from build123d import *

# Parameters (mm, degrees)
SKETCH8_R           = 1.6
SKETCH8_W           = 27.014473095
SKETCH8_H           = 14.822230288
SKETCH8_R_2         = 2.2
BOSS_EXTRUDE4_DEPTH = 8
SKETCH13_R          = 1.6
BOSS_EXTRUDE5_DEPTH = 3
CHAMFER1_SIZE       = 1
CHAMFER2_SIZE       = 0.5
CHAMFER3_SIZE       = 0.5
SKETCH14_W          = 50
SKETCH14_H          = 36
CUT_EXTRUDE1_DEPTH  = 6
CUT_EXTRUDE2_DEPTH  = 26


with BuildPart() as part:
    # Sketch8 → Boss-Extrude4 (new body)
    with BuildSketch(Plane(origin=(0, 0, 0), x_dir=(1, 0, 0), z_dir=(0, 1, 0))):
        with BuildLine():
            Line((57.021874501, 46.194423092), (3.021874501, 46.194423092))
            ThreePointArc((3.021874501, 46.194423092), (0.900554158, 45.315743435), (0.021874501, 43.194423092))
            Line((0.021874501, 43.194423092), (0.021874501, 3.194423092))
            ThreePointArc((0.021874501, 3.194423092), (0.900554158, 1.073102748), (3.021874501, 0.194423092))
            Line((3.021874501, 0.194423092), (57.021874501, 0.194423092))
            ThreePointArc((57.021874501, 0.194423092), (59.143194845, 1.073102748), (60.021874501, 3.194423092))
            Line((60.021874501, 3.194423092), (60.021874501, 43.194423092))
            ThreePointArc((60.021874501, 43.194423092), (59.143194845, 45.315743435), (57.021874501, 46.194423092))
        make_face()
        with Locations((30.021874501, 2.694423092)):
            Circle(SKETCH8_R, mode=Mode.SUBTRACT)
        with Locations((2.521874501, 23.194423092)):
            Circle(SKETCH8_R, mode=Mode.SUBTRACT)
        with Locations((30.021874501, 43.694423092)):
            Circle(SKETCH8_R, mode=Mode.SUBTRACT)
        Polygon((8.193945871, 28.957965299), (8.193945871, 41.194423092), (51.724223397, 41.194423092), (51.724223397, 37.388033247), (26.110307843, 37.388033247), (26.110307843, 28.957965299), align=None, mode=Mode.SUBTRACT)
        with Locations((41.514637954, 25.761884129)):
            Rectangle(SKETCH8_W, SKETCH8_H, mode=Mode.SUBTRACT)
        with Locations((22.240201254, 24.607965299)):
            Circle(SKETCH8_R_2, mode=Mode.SUBTRACT)
        with Locations((12.021874501, 24.607965299)):
            Circle(SKETCH8_R_2, mode=Mode.SUBTRACT)
    extrude(amount=BOSS_EXTRUDE4_DEPTH)

    # Sketch13 → Boss-Extrude5 (add)
    with BuildSketch(Plane(origin=(0, 8, 0), x_dir=(1, 0, 0), z_dir=(0, 1, 0))):
        with Locations((2.521874501, 23.194423092)):
            Circle(SKETCH13_R)
        with Locations((30.021874501, 2.694423092)):
            Circle(SKETCH13_R)
        with Locations((30.021874501, 43.694423092)):
            Circle(SKETCH13_R)
    extrude(amount=-BOSS_EXTRUDE5_DEPTH)

    # Chamfer1
    chamfer1_edges = [part.edges().sort_by_distance(p)[0] for p in [
        (59.143194845, 8, -1.073102748),
        (60.021874501, 8, -23.194423092),
        (59.143194845, 8, -45.315743435),
        (30.021874501, 8, -46.194423092),
        (0.900554158, 8, -45.315743435),
        (0.021874501, 8, -23.194423092),
        (0.900554158, 8, -1.073102748),
        (30.021874501, 8, -0.194423092),
    ]]
    chamfer(chamfer1_edges, length=CHAMFER1_SIZE)

    # Chamfer2
    chamfer2_edges = [part.edges().sort_by_distance(p)[0] for p in [
        (41.514637954, 8, -33.172999273),
        (55.021874501, 8, -25.761884129),
        (41.514637954, 8, -18.350768985),
        (28.007401406, 8, -25.761884129),
    ]]
    chamfer(chamfer2_edges, length=CHAMFER2_SIZE)

    # Chamfer3
    chamfer3_edges = [part.edges().sort_by_distance(p)[0] for p in [
        (20.040201254, 8, -24.607965299),
        (9.821874501, 8, -24.607965299),
    ]]
    chamfer(chamfer3_edges, length=CHAMFER3_SIZE)

    # Sketch14 → Cut-Extrude1 (cut)
    with BuildSketch(Plane.XZ):
        with Locations((30.021874501, -23.194423092)):
            Rectangle(SKETCH14_W, SKETCH14_H)
    extrude(amount=-CUT_EXTRUDE1_DEPTH, mode=Mode.SUBTRACT)

    # Sketch15 → Cut-Extrude2 (cut)
    with BuildSketch(Plane.ZY.offset(-26.110307843)):
        Polygon((-37.388033247, 7), (-34.086693064, 6), (-37.388033247, 6), align=None)
    extrude(amount=-CUT_EXTRUDE2_DEPTH, mode=Mode.SUBTRACT)


solid = part.part
The model under review builds one solid part; all positions refer to its coordinate system, in mm. A direction names the side the tool comes from. Round coordinates to 2 decimals unless told otherwise and drop trailing zeros. Loops run counter-clockwise (first coordinate to the right, second up) from the corner with the lowest first, then second, coordinate; pieces in that order, holes last. Notation, with made-up numbers: M 40.5,17 L 86.5,17 A30 ccw 86.5,43 Z; hole C -15.5,48 d11. An arc over 180 degrees is marked long. Answer as CSV lines item,"result".
1. To check wall thickness, follow L1, parallel to Z at x = 6.5, y = 3.75; L2, parallel to X at y = 4.75, z = -16.5; L3, parallel to X at y = 6.25, z = -37. State the ranges of each line that lie inside material, in increasing order. Write a range as [from, to].
Outcome:
L1,"z = [-46.19, -41.19], [-5.19, -0.19]"
L2,"x = [0.02, 5.02], [55.02, 60.02]"
L3,"x = [0.02, 8.19], [52.11, 60.02]"
2. We need section A-A (z = -38). Give the boundary of the cut face in (x, y).
Outcome:
outline,"M 0.02,0 L 5.02,0 L 5.02,6 L 8.19,6 L 8.19,8 L 1.02,8 L 0.02,7 Z; M 51.72,6 L 55.02,6 L 55.02,0 L 60.02,0 L 60.02,7 L 59.02,8 L 51.72,8 Z"
3. We need section C-C (x = 35). Give the boundary of the cut face in (y, z), plus the area to 3 significant figures.
Outcome:
outline,"M 0,-46.19 L 7,-46.19 L 8,-45.19 L 8,-41.19 L 0,-41.19 Z; M 0,-5.19 L 6,-5.19 L 6,-18.35 L 7.5,-18.35 L 8,-17.85 L 8,-1.19 L 7,-0.19 L 0,-0.19 Z; M 6,-34.09 L 7,-37.39 L 8,-37.39 L 8,-33.67 L 7.5,-33.17 L 6,-33.17 Z"
area,"112 mm2"
4. For faces 1 (the face through (32, 0, -42)), 2 (the face through (30, 5, -44)), 3 (the face through (51.724, 7, -39)), list the 3-axis set-ups (+Z, -Z, +X, -X, +Y, -Y) from which the entire face can be reached by the end or side of a thin tool; tool diameter is ignored.
Outcome:
face 1,"+Z, -Z, +X, -X, -Y"
face 2,"-Y"
face 3,"+Y, -Y"
5. We need section D-D (y = 3.5). Give the boundary of the cut face in (x, z), plus the area to 3 significant figures.
Outcome:
outline,"M 0.02,-43.19 A3 ccw 3.02,-46.19 L 57.02,-46.19 A3 ccw 60.02,-43.19 L 60.02,-3.19 A3 ccw 57.02,-0.19 L 3.02,-0.19 A3 ccw 0.02,-3.19 Z; hole C 2.52,-23.19 d3.2; hole M 5.02,-41.19 L 55.02,-41.19 L 55.02,-5.19 L 5.02,-5.19 Z; hole C 30.02,-43.69 d3.2; hole C 30.02,-2.69 d3.2"
area,"928 mm2"
6. We need section B-B (x = 54). Give the boundary of the cut face in (y, z).
Outcome:
outline,"M 0,-46.19 L 7,-46.19 L 8,-45.19 L 8,-33.67 L 7.5,-33.17 L 6,-33.17 L 6,-41.19 L 0,-41.19 Z; M 0,-5.19 L 6,-5.19 L 6,-18.35 L 7.5,-18.35 L 8,-17.85 L 8,-1.19 L 7,-0.19 L 0,-0.19 Z"
7. Insertion check: pin 1 Ø1 at (x, z) = (30.5, -3) entering from -Y. The pin has a flat end and moves straight along its axis. Give the tip position at first contact, or say it passes through.
Outcome:
pin 1,"stops at y = 5"
8. Draft analysis for pull direction X (two halves, no side actions). For faces 4 (the face through (0.924, 3.451, -45.339)), 5 (the face through (30, 3, -46.194)), 6 (the face through (13.205, 6.74, -26.463)), state which applies: pulls with the +X half, pulls with the -X half, needs draft (parallel to the pull), parting line crosses it, or undercut.
Outcome:
face 4,"pulls with the -X half"
face 5,"needs draft"
face 6,"undercut"
